Geometry: final body of the model. Coordinates: model frame, mm. A direction names the side the tool comes from. Round coordinates to 2 decimals unless told otherwise and drop trailing zeros. Order: outer loops, then holes, each group sorted by start corner. A loop starts at its lowest first (then second) coordinate and runs counter-clockwise, first axis right, second up. Notation, with made-up numbers: (19, 20.5) - (44, 20.5) arc R19 ccw to (44, 27.5) - close; hole circle Ø3 at (39.25, -34.75). An arc over 180 degrees is marked (long way). Put each result on its own line as item: value. Start each with the question number.
(1) Section D-D (y = 35.95). Output: boundary loops of the cut face in (x, z).
(2) Access query for faces 1 (the face through (-11, 20.95, 2)), 2 (the face through (20.946, 0.391, 1.972)), 3 (the face through (8, -25.95, 2)). Directions: +Z, -Z, +X, -X, +Y, -Y. A direction counts if a zero-diameter tool reaches every point of the face in a straight line with its end or side. Return the directions, or none.
(3) Pin query (flat end, axial travel): P1, Ø2.5, axis at x = 0, y = 35.95, coming from the +Z side; P2, Ø2, axis at y = 3.5, z = 2.5, coming from the -X side; P3, Ø2, axis at x = 2, z = 2, coming from the +Y side; P4, Ø1.2, axis at x = -10.5, z = 2, coming from the -Y side. Return the tip coordinate at first contact, or that it passes through.
(4) Material intervals for L1, parallel to Y at x = 0, z = 0.9; L2, parallel to Y at x = -14, z = 3.1; L3, parallel to X at y = 22, z = 3.6, sorted ascending. Write a range as [from, to].
(5) Section A-A (z = 2.9). Output: boundary loops of the cut face in (x, y), and give its area (3 significant figures).
(6) Section C-C (x = 3). Output: boundary loops of the cut face in (y, z).
(7) Section B-B (y = 25.95). Output: boundary loops of the cut face in (x, z), and give its area (3 significant figures).
(8) Pull-direction query (Y, two-part tool) for faces 4 (the face through (1.014, 38.773, 1.972)), 5 (the face through (16.838, -25.816, 1.972)), 6 (the face through (-3.63, -17.51, 1.97)); classes: released by +Y, released by -Y, zero draft, split by the parting line, or undercut.
from build123d import *

# Parameters (mm, degrees)
CROQUIS1_R              = 4
CROQUIS1_R_2            = 2.5
CROQUIS1_R_3            = 1.5
SALIENTE_EXTRUIR1_DEPTH = 4


with BuildPart() as part:
    # Croquis1 → Saliente-Extruir1 (new body)
    with BuildSketch(Plane.XY):
        with BuildLine():
            ThreePointArc((17.665369851, -25.41332737), (30.929543207, -1.1251031), (19.465124293, 24.062656467))
            Line((19.465124293, 24.062656467), (1.886764875, 38.28240612))
            ThreePointArc((1.886764875, 38.28240612), (1.000695169, 38.778181249), (0, 38.95))
            Line((0, 38.95), (-14, 38.95))
            ThreePointArc((-14, 38.95), (-15.75421382, 38.383666755), (-16.84611457, 36.898489248))
            Line((-16.84611457, 36.898489248), (-19.121320344, 30.071320344))
            ThreePointArc((-19.121320344, 30.071320344), (-19.771638598, 29.098050297), (-20, 27.95))
            Line((-20, 27.95), (-20, 23.95))
            ThreePointArc((-20, 23.95), (-19.121320344, 21.828679656), (-17, 20.95))
            Line((-17, 20.95), (-5, 20.95))
            ThreePointArc((-5, 20.95), (-0.298863721, 15.958939945), (4.964272191, 20.353341289))
            ThreePointArc((4.964272191, 20.353341289), (20.95, 0), (4.964272191, -20.353341289))
            ThreePointArc((4.964272191, -20.353341289), (-3.740540974, -17.632116153), (0, -25.95))
            Line((0, -25.95), (15.953056134, -25.95))
            ThreePointArc((15.953056134, -25.95), (16.85027904, -25.812689479), (17.665369851, -25.41332737))
        make_face()
        with Locations((0, -20.95)):
            Circle(CROQUIS1_R, mode=Mode.SUBTRACT)
        with Locations((0, 20.95)):
            Circle(CROQUIS1_R, mode=Mode.SUBTRACT)
        with Locations((-15, 25.95)):
            Circle(CROQUIS1_R_2, mode=Mode.SUBTRACT)
        with Locations((0, 35.95)):
            Circle(CROQUIS1_R_3, mode=Mode.SUBTRACT)
        with Locations((-14, 35.95)):
            Circle(CROQUIS1_R_3, mode=Mode.SUBTRACT)
    extrude(amount=SALIENTE_EXTRUIR1_DEPTH)


solid = part.part
Checks:
1. outline: (-17.16, 0) - (-15.5, 0) - (-15.5, 4) - (-17.16, 4) - close; (-12.5, 0) - (-1.5, 0) - (-1.5, 4) - (-12.5, 4) - close; (1.5, 0) - (4.77, 0) - (4.77, 4) - (1.5, 4) - close
2. face 1: +Z, -Z, -X, -Y
2. face 2: +Z, -Z
2. face 3: +Z, -Z, +X, -X, -Y
3. P1: passes through
3. P2: stops at x = 20.46
3. P3: stops at y = 38.78
3. P4: stops at y = 20.95
4. L1: y = [-25.95, -24.95], [-16.95, -15.95], [15.95, 16.95], [24.95, 34.45], [37.45, 38.95]
4. L2: y = [20.95, 23.66], [28.24, 34.45], [37.45, 38.95]
4. L3: x = [-19.28, -3.86], [3.86, 21.77]
5. outline: (-20, 23.95) arc R3 ccw to (-17, 20.95) - (-5, 20.95) arc R5 ccw to (4.96, 20.35) arc R20.95 cw to (4.96, -20.35) arc R5 ccw (long way) to (0, -25.95) - (15.95, -25.95) arc R3 ccw to (17.67, -25.41) arc R30.95 ccw to (19.47, 24.06) - (1.89, 38.28) arc R3 ccw to (0, 38.95) - (-14, 38.95) arc R3 ccw to (-16.85, 36.9) - (-19.12, 30.07) arc R3 ccw to (-20, 27.95) - close; hole circle Ø5 at (-15, 25.95); hole circle Ø3 at (-14, 35.95); hole circle Ø8 at (0, -20.95); hole circle Ø8 at (0, 20.95); hole circle Ø3 at (0, 35.95)
5. area: 1,120 mm²
6. outline: (-25.95, 0) - (-23.6, 0) - (-23.6, 4) - (-25.95, 4) - close; (-18.3, 0) - (-16.95, 0) - (-16.95, 4) - (-18.3, 4) - close; (16.95, 0) - (18.3, 0) - (18.3, 4) - (16.95, 4) - close; (23.6, 0) - (37.38, 0) - (37.38, 4) - (23.6, 4) - close
7. outline: (-20, 0) - (-17.5, 0) - (-17.5, 4) - (-20, 4) - close; (-12.5, 0) - (17.13, 0) - (17.13, 4) - (-12.5, 4) - close
7. area: 129 mm²
8. face 4: released by +Y
8. face 5: released by -Y
8. face 6: undercut
